Geometry: final body of the model. Coordinates: model frame, mm. Face numbers are marked on the shaded views. A direction names the side the tool comes from. Round coordinates to 2 decimals unless told otherwise and drop trailing zeros. Write each loop counter-clockwise with the first axis right and the second up, starting at its lowest first coordinate (ties: lowest second). Pieces come first, ordered by that corner, then holes. Notation, with made-up numbers: M -2.5,-27.75 L 6.5,-27.75 A30 cw 6.5,11.25 Z; hole C 21.25,-8 d11. An arc over 180 degrees is marked long. Use one line per item in the form item = value. Start each with the question number.
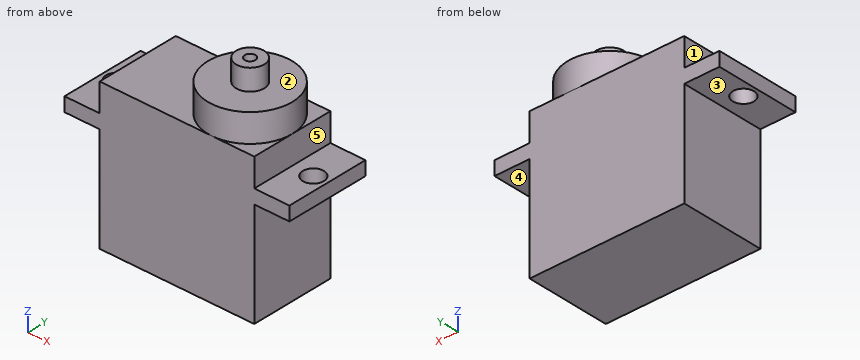
from build123d import *

# Parameters (mm, degrees)
CROQUIS1_W              = 32
CROQUIS1_H              = 12
SALIENTE_EXTRUIR1_DEPTH = 30
CROQUIS2_W              = 5
CROQUIS2_H              = 12
CORTAR_EXTRUIR1_DEPTH   = 15
CROQUIS3_W              = 32
CROQUIS3_H              = 12
CORTAR_EXTRUIR3_DEPTH   = 13
CROQUIS4_W              = 22
CROQUIS4_H              = 12
SALIENTE_EXTRUIR2_DEPTH = 4
CROQUIS5_R              = 6
SALIENTE_EXTRUIR3_DEPTH = 4
CROQUIS6_R              = 2
SALIENTE_EXTRUIR4_DEPTH = 3
CROQUIS7_R              = 0.75
CORTAR_EXTRUIR4_DEPTH   = 4
CROQUIS8_R              = 1.5
CORTAR_EXTRUIR5_DEPTH   = 4


with BuildPart() as part:
    # Croquis1 → Saliente-Extruir1 (new body)
    with BuildSketch(Plane.XY):
        Rectangle(CROQUIS1_W, CROQUIS1_H)
    extrude(amount=SALIENTE_EXTRUIR1_DEPTH)

    # Croquis2 → Cortar-Extruir1 (cut)
    with BuildSketch(Plane(origin=(0, 0, 0), x_dir=(-1, 0, 0), z_dir=(0, 0, -1))):
        with Locations((-13.5, 0)):
            Rectangle(CROQUIS2_W, CROQUIS2_H)
        with Locations((13.5, 0)):
            Rectangle(CROQUIS2_W, CROQUIS2_H)
    extrude(amount=-CORTAR_EXTRUIR1_DEPTH, mode=Mode.SUBTRACT)

    # Croquis3 → Cortar-Extruir3 (cut)
    with BuildSketch(Plane.XY.offset(30)):
        Rectangle(CROQUIS3_W, CROQUIS3_H)
    extrude(amount=-CORTAR_EXTRUIR3_DEPTH, mode=Mode.SUBTRACT)

    # Croquis4 → Saliente-Extruir2 (add)
    with BuildSketch(Plane.XY.offset(17)):
        Rectangle(CROQUIS4_W, CROQUIS4_H)
    extrude(amount=SALIENTE_EXTRUIR2_DEPTH)

    # Croquis5 → Saliente-Extruir3 (add)
    with BuildSketch(Plane.XY.offset(21)):
        with Locations((5, 0)):
            Circle(CROQUIS5_R)
    extrude(amount=SALIENTE_EXTRUIR3_DEPTH)

    # Croquis6 → Saliente-Extruir4 (add)
    with BuildSketch(Plane.XY.offset(25)):
        with Locations((5, 0)):
            Circle(CROQUIS6_R)
    extrude(amount=SALIENTE_EXTRUIR4_DEPTH)

    # Croquis7 → Cortar-Extruir4 (cut)
    with BuildSketch(Plane.XY.offset(28)):
        with Locations((5, 0)):
            Circle(CROQUIS7_R)
    extrude(amount=-CORTAR_EXTRUIR4_DEPTH, mode=Mode.SUBTRACT)

    # Croquis8 → Cortar-Extruir5 (cut)
    with BuildSketch(Plane.XY.offset(17)):
        with Locations((-14, 0)):
            Circle(CROQUIS8_R)
    cortar_extruir5 = extrude(amount=-CORTAR_EXTRUIR5_DEPTH, mode=Mode.SUBTRACT)

    # Simetría1: Cortar-Extruir5 across plane
    add(cortar_extruir5.mirror(Plane(origin=(0, 0, 0), x_dir=(0, 0, 1), z_dir=(1, 0, 0))), mode=Mode.SUBTRACT)


solid = part.part
1. Contact query for flat-ended pins moving along their axis: pin 1 (5 mm diameter, centred on y = -3, z = 24.5, fed in from +X); pin 2 (3 mm diameter, centred on y = -3.5, z = 21, fed in from -X); pin 3 (1.5 mm diameter, centred on x = -13, y = -0.5, fed in from +Z). Output: stop coordinate, or through.
2. Section query D-D (y = 2.75). Return loops of the section in (x, z).
3. Ray query, probe 1 along Y at (x, z) = (-14, 15.6); probe 2 along Y at (x, z) = (5, 26.75); probe 3 along X at (y, z) = (4.25, 6.5). Return the intervals inside material, ascending.
4. Section query A-A (x = 14). Return loops of the section in (y, z), then the cut area to 3 significant figures.
5. Section query C-C (z = 9). Return loops of the section in (x, y).
6. Set-up query: the marked faces 1, 2, 3, 4 and 5. Return all of +Z, -Z, +X, -X, +Y, -Y with unobstructed straight access to the full face (end or side cutting, diameter ignored); none if empty.
7. Section query B-B (y = -5). Return loops of the section in (x, z), then the cut area to 3 significant figures.
Checks:
q1.pin_1 = 10.98
q1.pin_2 = -11
q1.pin_3 = 17
q2.outline = M -16,15 L -11,15 L -11,0 L 11,0 L 11,15 L 16,15 L 16,17 L 11,17 L 11,21 L 10.33,21 L 10.33,25 L -0.33,25 L -0.33,21 L -11,21 L -11,17 L -16,17 Z
q3.probe_1 = -6 to -1.5, 1.5 to 6
q3.probe_2 = -2 to -0.75, 0.75 to 2
q3.probe_3 = -11 to 11
q4.outline = M -6,15 L -1.5,15 L -1.5,17 L -6,17 Z; M 1.5,15 L 6,15 L 6,17 L 1.5,17 Z
q4.area = 18.0 mm^2
q5.outline = M -11,-6 L 11,-6 L 11,6 L -11,6 Z
q6.face_1 = +Z, -X, +Y, -Y
q6.face_2 = +Z
q6.face_3 = -Z, -X, +Y, -Y
q6.face_4 = -Z, +X, +Y, -Y
q6.face_5 = +Z, +X, +Y, -Y
q7.outline = M -16,15 L -11,15 L -11,0 L 11,0 L 11,15 L 16,15 L 16,17 L 11,17 L 11,21 L 8.32,21 L 8.32,25 L 1.68,25 L 1.68,21 L -11,21 L -11,17 L -16,17 Z
q7.area = 509 mm^2
